Input: part model. Units: mm. Frame: model coordinates. Round coordinates to 2 decimals unless told otherwise and drop trailing zeros. Write each loop counter-clockwise with the first axis right and the second up, starting at its lowest first coordinate (ties: lowest second). Pieces come first, ordered by that corner, then holes. Notation, with made-up numbers: (2.5, 66.5) - (36.5, 66.5) arc R18 cw to (36.5, 100.5) - close; hole circle Ø2 at (41, 23). An arc over 180 degrees is marked (long way). Use one line per item in the form item = value.
```python
from build123d import *

# Parameters (mm, degrees)
F0_R     = 37.5
F1_DEPTH = 12.5
F2_W     = 3
F2_H     = 3
F3_DEPTH = 12.5
F4_R     = 1.5


with BuildPart() as f1:
    # F0 (on Front) → F1 (new body)
    with BuildSketch(Plane.XZ):
        Circle(F0_R)
    extrude(amount=F1_DEPTH)

    # F2 (on face) → F3 (cut, through all)
    with BuildSketch(Plane(origin=(0, 0, 0), x_dir=(-1, 0, 0), z_dir=(0, 1, 0))):
        Rectangle(F2_W, F2_H)
    extrude(amount=-F3_DEPTH, mode=Mode.SUBTRACT)

    # F4
    f4_edges = [f1.edges().sort_by_distance(p)[0] for p in [
        (-37.5, 0, 0),
        (-37.5, -12.5, 0),
    ]]
    fillet(f4_edges, radius=F4_R)


solid = f1.part
```
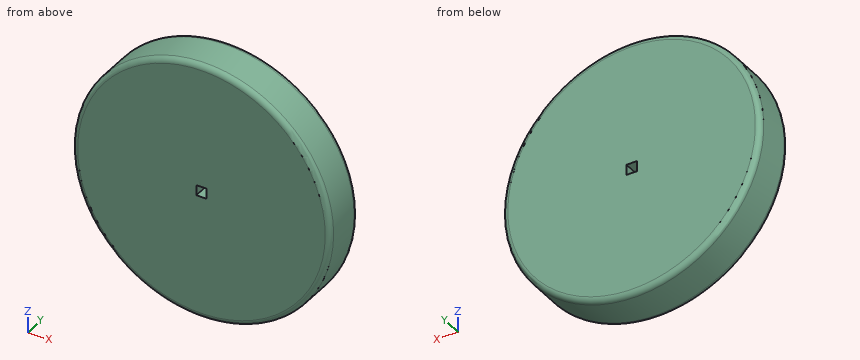
(1) Cut plane A-A on z = 0. Output: boundary loops of the cut face in (x, y), then the cut area to 3 significant figures.
Derived:
outline = (-37.5, -11) arc R1.5 ccw to (-36, -12.5) - (-1.5, -12.5) - (-1.5, 0) - (-36, 0) arc R1.5 ccw to (-37.5, -1.5) - close; (1.5, -12.5) - (36, -12.5) arc R1.5 ccw to (37.5, -11) - (37.5, -1.5) arc R1.5 ccw to (36, 0) - (1.5, 0) - close
area = 898 mm^2
(2) Material intervals for L1, parallel to X at y = -11.75, z = -8.5; L2, parallel to X at y = -1.25, z = -1; L3, parallel to X at y = -5.75, z = 25.5, sorted ascending.
Derived:
L1 = -36.32 to 36.32
L2 = -37.47 to -1.5, 1.5 to 37.47
L3 = -27.5 to 27.5
(3) Cut plane C-C on y = -3.5. Output: boundary loops of the cut face in (x, z).
Derived:
outline = circle Ø75 at (0, 0); hole (-1.5, -1.5) - (1.5, -1.5) - (1.5, 1.5) - (-1.5, 1.5) - close
(4) Cut plane B-B on x = 0. Output: boundary loops of the cut face in (y, z).
Derived:
outline = (-12.5, -36) arc R1.5 ccw to (-11, -37.5) - (-1.5, -37.5) arc R1.5 ccw to (0, -36) - (0, -1.5) - (-12.5, -1.5) - close; (-12.5, 1.5) - (0, 1.5) - (0, 36) arc R1.5 ccw to (-1.5, 37.5) - (-11, 37.5) arc R1.5 ccw to (-12.5, 36) - close
(5) First-contact query: pin 1 Ø2 at (x, y) = (-23.5, -2.5) entering from +Z; pin 2 Ø1.5 at (x, y) = (0, -7) entering from +Z; pin 3 Ø1 at (x, z) = (-23, -25) entering from +Y; pin 4 Ø1 at (x, y) = (18, -2.5) entering from +Z. Flat tips, straight axial feed; report the tip coordinate or a pass-through.
Derived:
pin_1 = 30
pin_2 = 37.5
pin_3 = 0
pin_4 = 33.17
